The model under review builds one solid part; all positions refer to its coordinate system, in mm. A direction names the side the tool comes from. Coordinates: 2 decimals unless noted, no trailing zeros. Loops run counter-clockwise (first coordinate to the right, second up) from the corner with the lowest first, then second, coordinate; pieces in that order, holes last. Notation, with made-up numbers: (26, 63) - (59, 63) arc R28 cw to (59, 87) - close; hole circle Ø2 at (25, 44). An arc over 180 degrees is marked (long way). Use a Markdown table: item, result. Add a question column.
1) For faces 4 (the flat face through (-15, 6, 14)), 5 (the flat face through (-1, 46.9, 7)), 6 (the flat face through (-3.015, -40.608, 1.578)), 7 (the flat face through (30, -5, 14)), list the 3-axis set-ups (+Z, -Z, +X, -X, +Y, -Y) from which the entire face can be reached by the end or side of a thin tool; tool diameter is ignored.
2) Add section A-A, the plane z = 8.5. Give the number of separate pieces and of enclosed holes in the cut face, and give its area (3 significant figures).
3) To check wall thickness, follow L1, parallel to Y at x = -25, z = 4.25; L2, parallel to X at y = -29.5, z = 3; L3, parallel to Y at x = 32, z = 6.5. State the ranges of each line that lie inside material, in increasing order. Write a range as [from, to].
4) The part is to be moulded in two halves that separate along X. For faces 1 (the cylindrical face through (-0.923, -40.674, 9.017)), 2 (the cylindrical face through (30.103, 10.581, -1.426)), 3 (the flat face through (20, -7, 14)), say which applies: pulls with the +X half, pulls with the -X half, needs draft (parallel to the pull), parting line crosses it, or undercut.
5) Clearance check with flat-ended pins moving along their axes: pin 1 (4 mm diameter, centred on x = -8.5, y = -7.5, fed in from -Z); pin 2 (1 mm diameter, centred on x = 17, y = -26.5, fed in from -Z); pin 3 (0.8 mm diameter, centred on x = 33, y = -6.5, fed in from +Z). State where each tip first meets the part, or that it passes through.
6) Add section D-D, the plane x = -13. Give the boundary of the cut face in (y, z).
```python
from build123d import *

# Parameters (mm, degrees)
SKETCH1_W           = 80
SKETCH1_H           = 93.8
BOSS_EXTRUDE1_DEPTH = 15
SKETCH2_W           = 10
SKETCH2_H           = 15
CUT_EXTRUDE1_DEPTH  = 10
SKETCH3_R           = 2
CUT_EXTRUDE2_DEPTH  = 94.939395357
SKETCH4_W           = 20
SKETCH4_H           = 25
SKETCH4_W_2         = 10
SKETCH4_H_2         = 15
BOSS_EXTRUDE2_DEPTH = 5
FILLET1_R           = 5
SKETCH5_R           = 2
CUT_EXTRUDE3_DEPTH  = 2.5
SKETCH6_W           = 3
SKETCH6_H           = 3
CUT_EXTRUDE4_DEPTH  = 94.939395357
SKETCH7_R           = 2
CUT_EXTRUDE5_DEPTH  = 3.2
SKETCH8_R           = 2
CUT_EXTRUDE6_DEPTH  = 64.439813997
CUT_EXTRUDE7_REACH  = 66.804
SKETCH9_W           = 10.4
SKETCH9_H           = 15.4
SKETCH10_R          = 3.5
CUT_EXTRUDE8_DEPTH  = 4
SKETCH11_R          = 2
CUT_EXTRUDE9_DEPTH  = 64.439813997
FILLET3_R           = 1
SKETCH12_W          = 5
SKETCH12_H          = 20
BOSS_EXTRUDE4_DEPTH = 5


with BuildPart() as part:
    # Sketch1 → Boss-Extrude1 (new body)
    with BuildSketch(Plane.XY):
        Rectangle(SKETCH1_W, SKETCH1_H)
    extrude(amount=BOSS_EXTRUDE1_DEPTH)

    # Sketch2 → Cut-Extrude1 (cut)
    with BuildSketch(Plane(origin=(0, 0, 0), x_dir=(-1, 0, 0), z_dir=(0, 0, -1))):
        with Locations((30, -24.4)):
            Rectangle(SKETCH2_W, SKETCH2_H)
        with Locations((-30, -24.4)):
            Rectangle(SKETCH2_W, SKETCH2_H)
        with Locations((30, 24.584880812)):
            Rectangle(SKETCH2_W, SKETCH2_H)
        with Locations((-30, 24.584880812)):
            Rectangle(SKETCH2_W, SKETCH2_H)
    extrude(amount=-CUT_EXTRUDE1_DEPTH, mode=Mode.SUBTRACT)

    # Sketch3 → Cut-Extrude2 (cut, through all)
    with BuildSketch(Plane(origin=(40, 0, 0), x_dir=(0, 0, -1), z_dir=(1, 0, 0))):
        with Locations((-5, 24.584880812)):
            Circle(SKETCH3_R)
        with Locations((-5, -24.4)):
            Circle(SKETCH3_R)
    extrude(amount=-CUT_EXTRUDE2_DEPTH, mode=Mode.SUBTRACT)

    # Sketch4 → Boss-Extrude2 (add)
    # profile 1 of 4: a face of its own
    with BuildSketch(Plane(origin=(0, 0, 0), x_dir=(-1, 0, 0), z_dir=(0, 0, -1))):
        with Locations((-30, 24.584880812)):
            Rectangle(SKETCH4_W, SKETCH4_H)
        with Locations((-30, 24.584880812)):
            Rectangle(SKETCH4_W_2, SKETCH4_H_2, mode=Mode.SUBTRACT)
    # profile 2 of 4: a face of its own
    with BuildSketch(Plane(origin=(0, 0, 0), x_dir=(-1, 0, 0), z_dir=(0, 0, -1))):
        with Locations((30, 24.584880812)):
            Rectangle(SKETCH4_W, SKETCH4_H)
        with Locations((30, 24.584880812)):
            Rectangle(SKETCH4_W_2, SKETCH4_H_2, mode=Mode.SUBTRACT)
    # profile 3 of 4: a face of its own
    with BuildSketch(Plane(origin=(0, 0, 0), x_dir=(-1, 0, 0), z_dir=(0, 0, -1))):
        with Locations((30, -24.584880812)):
            Rectangle(SKETCH4_W, SKETCH4_H)
        with Locations((30, -24.584880812)):
            Rectangle(SKETCH4_W_2, SKETCH4_H_2, mode=Mode.SUBTRACT)
    # profile 4 of 4: a face of its own
    with BuildSketch(Plane(origin=(0, 0, 0), x_dir=(-1, 0, 0), z_dir=(0, 0, -1))):
        with Locations((-30, -24.584880812)):
            Rectangle(SKETCH4_W, SKETCH4_H)
        with Locations((-30, -24.584880812)):
            Rectangle(SKETCH4_W_2, SKETCH4_H_2, mode=Mode.SUBTRACT)
    extrude(amount=BOSS_EXTRUDE2_DEPTH)

    # Fillet1
    fillet1_edges = [part.edges().sort_by_distance(p)[0] for p in [
        (-30, -37.084880812, 0),
        (30, -37.084880812, 0),
        (-30, -12.084880812, 0),
        (30, -12.084880812, 0),
        (-30, 37.084880812, 0),
        (30, 37.084880812, 0),
        (-30, 12.084880812, 0),
        (30, 12.084880812, 0),
        (20, 24.584880812, 0),
        (-20, 24.584880812, 0),
        (-20, -24.584880812, 0),
        (20, -24.584880812, 0),
    ]]
    fillet(fillet1_edges, radius=FILLET1_R - 0.0001)  # a hair under: the kernel refuses the full size

    # Sketch5 → Cut-Extrude3 (cut)
    with BuildSketch(Plane(origin=(0, 0, 0), x_dir=(-1, 0, 0), z_dir=(0, 0, -1))):
        with Locations((0, -26.9)):
            Circle(SKETCH5_R)
        with Locations((0, 27.08)):
            Circle(SKETCH5_R)
    extrude(amount=-CUT_EXTRUDE3_DEPTH, mode=Mode.SUBTRACT)

    # Sketch6 → Cut-Extrude4 (cut, through all)
    with BuildSketch(Plane(origin=(40, 0, 0), x_dir=(0, 0, -1), z_dir=(1, 0, 0))):
        with Locations((-13.5, 6.5)):
            Rectangle(SKETCH6_W, SKETCH6_H)
        with Locations((-13.5, -6.5)):
            Rectangle(SKETCH6_W, SKETCH6_H)
    extrude(amount=-CUT_EXTRUDE4_DEPTH, mode=Mode.SUBTRACT)

    # Sketch7 → Cut-Extrude5 (cut)
    # profile 1 of 4: a face of its own
    with BuildSketch(Plane(origin=(0, 0, 0), x_dir=(-1, 0, 0), z_dir=(0, 0, -1))):
        Polygon((-2.000518683, -42.365), (-4.001037365, -38.9), (-2.000518683, -35.435), (2.000518683, -35.435), (4.001037365, -38.9), (2.000518683, -42.365), align=None)
        with Locations(Location((0, -38.9, 0), (0, 0, 180))):
            Circle(SKETCH7_R, mode=Mode.SUBTRACT)
    # profile 2 of 4: a face of its own
    with BuildSketch(Plane(origin=(0, 0, 0), x_dir=(-1, 0, 0), z_dir=(0, 0, -1))):
        Polygon((28.004736137, 0), (30.002368069, -3.46), (33.997631931, -3.46), (35.995263863, 0), (33.997631931, 3.46), (30.002368069, 3.46), align=None)
        with Locations((32, 0)):
            Circle(SKETCH7_R, mode=Mode.SUBTRACT)
    # profile 3 of 4: a face of its own
    with BuildSketch(Plane(origin=(0, 0, 0), x_dir=(-1, 0, 0), z_dir=(0, 0, -1))):
        Polygon((-4.001037365, 38.9), (-2.000518683, 35.435), (2.000518683, 35.435), (4.001037365, 38.9), (2.000518683, 42.365), (-2.000518683, 42.365), align=None)
        with Locations((0, 38.9)):
            Circle(SKETCH7_R, mode=Mode.SUBTRACT)
    # profile 4 of 4: a face of its own
    with BuildSketch(Plane(origin=(0, 0, 0), x_dir=(-1, 0, 0), z_dir=(0, 0, -1))):
        Polygon((-30.002368069, 3.46), (-28.004736137, 0), (-30.002368069, -3.46), (-33.997631931, -3.46), (-35.995263863, 0), (-33.997631931, 3.46), align=None)
        with Locations(Location((-32, 0, 0), (0, 0, 180))):
            Circle(SKETCH7_R, mode=Mode.SUBTRACT)
    extrude(amount=-CUT_EXTRUDE5_DEPTH, mode=Mode.SUBTRACT)

    # Sketch8 → Cut-Extrude6 (cut, through all)
    with BuildSketch(Plane(origin=(0, 0, 0), x_dir=(-1, 0, 0), z_dir=(0, 0, -1))):
        with Locations((-32, 0)):
            Circle(SKETCH8_R)
        with Locations((0, -38.9)):
            Circle(SKETCH8_R)
        with Locations((32, 0)):
            Circle(SKETCH8_R)
        with Locations((0, 38.9)):
            Circle(SKETCH8_R)
    extrude(amount=-CUT_EXTRUDE6_DEPTH, mode=Mode.SUBTRACT)

    # Cut-Extrude7: up to this face of the body (flat: up to its plane)
    cut_extrude7_end = Plane(part.part.faces().sort_by_distance((30, 24.584880812, 10))[0])
    # Sketch9 → Cut-Extrude7 (cut, up to the picked face)
    with BuildSketch(Plane(origin=(0, 0, -5), x_dir=(-1, 0, 0), z_dir=(0, 0, -1)), mode=Mode.PRIVATE) as cut_extrude7_sk1:
        with Locations((-30, 24.584880812)):
            Rectangle(SKETCH9_W, SKETCH9_H)
    cut_extrude7_tool1 = split(extrude(cut_extrude7_sk1.sketch, amount=-CUT_EXTRUDE7_REACH, mode=Mode.PRIVATE), bisect_by=cut_extrude7_end, keep=Keep.BOTH, mode=Mode.PRIVATE)
    # Sketch9 → Cut-Extrude7 (cut, up to the picked face)
    with BuildSketch(Plane(origin=(0, 0, -5), x_dir=(-1, 0, 0), z_dir=(0, 0, -1)), mode=Mode.PRIVATE) as cut_extrude7_sk2:
        with Locations((30, 24.584880812)):
            Rectangle(SKETCH9_W, SKETCH9_H)
    cut_extrude7_tool2 = split(extrude(cut_extrude7_sk2.sketch, amount=-CUT_EXTRUDE7_REACH, mode=Mode.PRIVATE), bisect_by=cut_extrude7_end, keep=Keep.BOTH, mode=Mode.PRIVATE)
    # Sketch9 → Cut-Extrude7 (cut, up to the picked face)
    with BuildSketch(Plane(origin=(0, 0, -5), x_dir=(-1, 0, 0), z_dir=(0, 0, -1)), mode=Mode.PRIVATE) as cut_extrude7_sk3:
        with Locations((30, -24.584880812)):
            Rectangle(SKETCH9_W, SKETCH9_H)
    cut_extrude7_tool3 = split(extrude(cut_extrude7_sk3.sketch, amount=-CUT_EXTRUDE7_REACH, mode=Mode.PRIVATE), bisect_by=cut_extrude7_end, keep=Keep.BOTH, mode=Mode.PRIVATE)
    # Sketch9 → Cut-Extrude7 (cut, up to the picked face)
    with BuildSketch(Plane(origin=(0, 0, -5), x_dir=(-1, 0, 0), z_dir=(0, 0, -1)), mode=Mode.PRIVATE) as cut_extrude7_sk4:
        with Locations((-30, -24.584880812)):
            Rectangle(SKETCH9_W, SKETCH9_H)
    cut_extrude7_tool4 = split(extrude(cut_extrude7_sk4.sketch, amount=-CUT_EXTRUDE7_REACH, mode=Mode.PRIVATE), bisect_by=cut_extrude7_end, keep=Keep.BOTH, mode=Mode.PRIVATE)
    add(cut_extrude7_tool1.solids().sort_by(Axis((30, 24.584881, -5), (0, 0, 1)))[0], mode=Mode.SUBTRACT)
    add(cut_extrude7_tool2.solids().sort_by(Axis((-30, 24.584881, -5), (0, 0, 1)))[0], mode=Mode.SUBTRACT)
    add(cut_extrude7_tool3.solids().sort_by(Axis((-30, -24.584881, -5), (0, 0, 1)))[0], mode=Mode.SUBTRACT)
    add(cut_extrude7_tool4.solids().sort_by(Axis((30, -24.584881, -5), (0, 0, 1)))[0], mode=Mode.SUBTRACT)

    # Sketch10 → Cut-Extrude8 (cut)
    with BuildSketch(Plane(origin=(0, 0, 0), x_dir=(-1, 0, 0), z_dir=(0, 0, -1))):
        Circle(SKETCH10_R)
    extrude(amount=-CUT_EXTRUDE8_DEPTH, mode=Mode.SUBTRACT)

    # Sketch11 → Cut-Extrude9 (cut, through all)
    with BuildSketch(Plane(origin=(0, 0, 0), x_dir=(-1, 0, 0), z_dir=(0, 0, -1))):
        Circle(SKETCH11_R)
    extrude(amount=-CUT_EXTRUDE9_DEPTH, mode=Mode.SUBTRACT)

    # Fillet3
    fillet3_edges = [part.edges().sort_by_distance(p)[0] for p in [
        (0, 8, 12),
        (0, 5, 12),
        (0, -5, 12),
        (0, -8, 12),
    ]]
    fillet(fillet3_edges, radius=FILLET3_R)

    # Sketch12 → Boss-Extrude4 (add)
    with BuildSketch(Plane.XY.offset(15)):
        with Locations((-17.5, -0.1)):
            Rectangle(SKETCH12_W, SKETCH12_H)
        with Locations((17.5, -0.1)):
            Rectangle(SKETCH12_W, SKETCH12_H)
    extrude(amount=-BOSS_EXTRUDE4_DEPTH)


solid = part.part
```
From the geometry:
| question | item | result |
|---|---|---|
| 1 | face 4 | +Z |
| 1 | face 5 | +Z, -Z, +X, -X, +Y |
| 1 | face 6 | -Z |
| 1 | face 7 | +Z, +X |
| 2 | separate pieces | 1 |
| 2 | enclosed holes | 9 |
| 2 | area | 6,800 mm^2 |
| 3 | L1 | y = [-46.9, -32.28], [-16.88, 16.88], [32.28, 46.9] |
| 3 | L2 | x = [-40, -35.2], [-24.8, 24.8], [35.2, 40] |
| 3 | L3 | y = [-46.9, -32.28], [-16.88, -2], [2, 16.88], [32.28, 46.9] |
| 4 | face 1 | undercut |
| 4 | face 2 | needs draft |
| 4 | face 3 | pulls with the +X half |
| 5 | pin 1 | stops at z = 0 |
| 5 | pin 2 | stops at z = -0.67 |
| 5 | pin 3 | stops at z = 12 |
| 6 | outline | (-46.9, 0) - (46.9, 0) - (46.9, 15) - (8, 15) - (8, 13) arc R1 cw to (7, 12) - (6, 12) arc R1 cw to (5, 13) - (5, 15) - (-5, 15) - (-5, 13) arc R1 cw to (-6, 12) - (-7, 12) arc R1 cw to (-8, 13) - (-8, 15) - (-46.9, 15) - close; hole circle Ø4 at (-24.4, 5); hole circle Ø4 at (24.58, 5) |
